```python
from build123d import *

# Parameters (mm, degrees)
CROQUIS1_W              = 16
CROQUIS1_H              = 23
SALIENTE_EXTRUIR1_DEPTH = 2
CROQUIS2_W              = 13
CROQUIS2_H              = 20
SALIENTE_EXTRUIR2_DEPTH = 10
SALIENTE_EXTRUIR3_DEPTH = 6.5
CROQUIS4_R              = 2
CROQUIS4_R_2            = 1.5
CROQUIS4_W              = 4
CROQUIS4_H              = 1
CORTAR_EXTRUIR1_DEPTH   = 0.6
SALIENTE_EXTRUIR6_DEPTH = 6.5
REDONDEO1_R             = 0.5
CROQUIS6_R              = 0.75
SALIENTE_EXTRUIR7_DEPTH = 0.25
MATRIZL1_COUNT          = 2
MATRIZL1_PITCH          = 6.666666667
MATRIZL2_COUNT          = 2
MATRIZL2_PITCH          = 6.666666667


with BuildPart() as part:
    # Croquis1 → Saliente-Extruir1 (new body)
    with BuildSketch(Plane(origin=(0, 0, 0), x_dir=(1, 0, 0), z_dir=(0, 1, 0))):
        Rectangle(CROQUIS1_W, CROQUIS1_H)
    extrude(amount=SALIENTE_EXTRUIR1_DEPTH)

    # Croquis2 → Saliente-Extruir2 (add)
    with BuildSketch(Plane.XZ):
        Rectangle(CROQUIS2_W, CROQUIS2_H)
    extrude(amount=SALIENTE_EXTRUIR2_DEPTH)

    # Croquis3 → Saliente-Extruir3 (add, symmetric)
    with BuildSketch(Plane(origin=(0, 0, 0), x_dir=(0, 0, -1), z_dir=(1, 0, 0))):
        with BuildLine():
            Line((8.5, 2), (-8.5, 2))
            Line((-8.5, 2), (-0.603629693, 3.914367561))
            ThreePointArc((-0.603629693, 3.914367561), (0.234425411, 4.156697965), (1.048170976, 4.471147542))
            Line((1.048170976, 4.471147542), (5.618369194, 6.470445319))
            ThreePointArc((5.618369194, 6.470445319), (5.795753126, 6.511830798), (5.976190969, 6.486930957))
            Line((5.976190969, 6.486930957), (6.048439126, 6.462964543))
            ThreePointArc((6.048439126, 6.462964543), (7.345603515, 5.609203874), (8.042100494, 4.221243251))
            Line((8.042100494, 4.221243251), (8.5, 2))
        make_face()
    extrude(amount=SALIENTE_EXTRUIR3_DEPTH, both=True)

    # Croquis4 → Cortar-Extruir1 (cut)
    with BuildSketch(Plane(origin=(0, 4.265025315, 1.351360717), x_dir=(1, 0, 0), z_dir=(0, 0.95329272, 0.302047992))):
        with Locations((0, 4)):
            Circle(CROQUIS4_R)
        with Locations((0, 4)):
            Circle(CROQUIS4_R_2, mode=Mode.SUBTRACT)
        with Locations((0, -4)):
            Rectangle(CROQUIS4_W, CROQUIS4_H)
    extrude(amount=-CORTAR_EXTRUIR1_DEPTH, mode=Mode.SUBTRACT)

    # Croquis5 → Saliente-Extruir6 (add, symmetric)
    with BuildSketch(Plane(origin=(0, 0, 0), x_dir=(0, 0, -1), z_dir=(1, 0, 0))):
        Polygon((-10, -0.2), (-10.3, -0.2), (-10.3, -0.5), (-10.6, -0.5), (-10.6, -0.8), (-10.9, -0.8), (-10, -10), (-10, -8), (-10.6, -1.1), (-10.3, -1.1), (-10.3, -0.8), (-10, -0.8), align=None)
    saliente_extruir6 = extrude(amount=SALIENTE_EXTRUIR6_DEPTH, both=True)

    # Simetría2: Saliente-Extruir6 across plane
    add(saliente_extruir6.mirror(Plane.XY))

    # Redondeo1
    redondeo1_edges = [part.edges().sort_by_distance(p)[0] for p in [
        (-8, 1, -11.5),
        (8, 1, -11.5),
        (8, 1, 11.5),
        (-8, 1, 11.5),
    ]]
    fillet(redondeo1_edges, radius=REDONDEO1_R)

    # Croquis6 → Saliente-Extruir7 (add, symmetric)
    with BuildSketch(Plane.XY):
        with BuildLine():
            Line((2.5, -10), (-2.5, -10))
            Line((-2.5, -10), (-2.5, -15.826794919))
            ThreePointArc((-2.5, -15.826794919), (-2.459807621, -15.976794919), (-2.35, -16.08660254))
            Line((-2.35, -16.08660254), (-0.65, -17.068097998))
            ThreePointArc((-0.65, -17.068097998), (-0.540192379, -17.177905619), (-0.5, -17.327905619))
            Line((-0.5, -17.327905619), (-0.5, -17.354700538))
            ThreePointArc((-0.5, -17.354700538), (-0.412132034, -17.566832573), (-0.2, -17.654700538))
            Line((-0.2, -17.654700538), (0.2, -17.654700538))
            ThreePointArc((0.2, -17.654700538), (0.412132034, -17.566832573), (0.5, -17.354700538))
            Line((0.5, -17.354700538), (0.5, -17.327905619))
            ThreePointArc((0.5, -17.327905619), (0.540192379, -17.177905619), (0.65, -17.068097998))
            Line((0.65, -17.068097998), (2.35, -16.08660254))
            ThreePointArc((2.35, -16.08660254), (2.459807621, -15.976794919), (2.5, -15.826794919))
            Line((2.5, -15.826794919), (2.5, -10))
        make_face()
        with Locations((0, -15.154700538)):
            Circle(CROQUIS6_R, mode=Mode.SUBTRACT)
    saliente_extruir7 = extrude(amount=SALIENTE_EXTRUIR7_DEPTH, both=True)

    # MatrizL1: Saliente-Extruir7 ×2
    with Locations(*[(0, 0, -i * MATRIZL1_PITCH) for i in range(1, MATRIZL1_COUNT)]):
        add(saliente_extruir7)

    # MatrizL2: Saliente-Extruir7 ×2
    with Locations(*[(0, 0, i * MATRIZL2_PITCH) for i in range(1, MATRIZL2_COUNT)]):
        add(saliente_extruir7)


solid = part.part
```
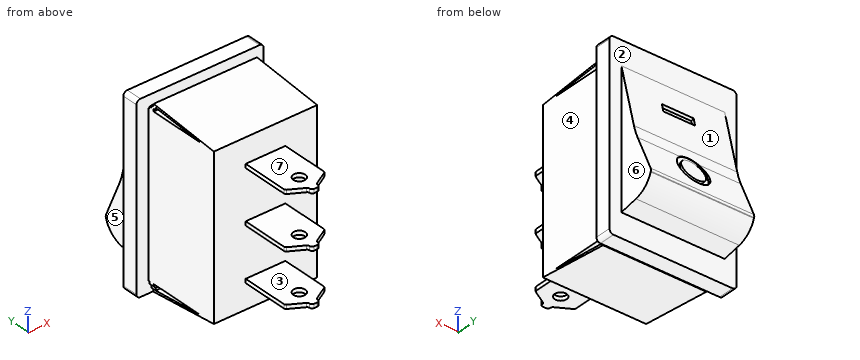
Check sheet for the modelled part. Datum: model origin and axes. Units: mm. Face numbers are marked on the shaded views. A direction names the side the tool comes from. Round coordinates to 2 decimals unless told otherwise and drop trailing zeros. Order: outer loops, then holes, each group sorted by start corner. A loop starts at its lowest first (then second) coordinate and runs counter-clockwise, first axis right, second up.
1) Go/stop test with flat-tipped pins: pin 1 Ø10 at (y, z) = (-8, -1) entering from -X; pin 2 Ø0.6 at (y, z) = (-14.5, 0) entering from +X; pin 3 Ø2 at (y, z) = (-12, 4.5) entering from +X; pin 4 Ø5 at (x, y) = (3.5, -11.5) entering from -Z. Record where each tip stops, or that it passes through.
2) Scan lines: line 1 (Z direction, x = 1.5, y = -11.75); line 2 (Y direction, x = 6.75, z = 3.25); line 3 (Z direction, x = -1.25, y = -5.75). Record each from-to range of solid material in increasing order.
3) Section check A-A (z = -9.25). Record the boundary of the cut face in (x, y).
4) Mould release check, pull along Z, two halves, no side actions. Record for the marked faces 1, 2 and 3: +Z half, -Z half, draft (parallel to the pull), parting line (faces both ways), or undercut.
5) Tool access check on the marked faces 4, 5, 6 and 7. Record the directions out of +Z, -Z, +X, -X, +Y, -Y that give a thin tool (end or side, any length) a straight path to the whole face; none if there is none.
Result:
1. pin 1: stops at x = -6.5
1. pin 2: stops at x = 2.5
1. pin 3: passes through
1. pin 4: stops at z = -10.1
2. line 1: z = -6.92 to -6.42, -0.25 to 0.25, 6.42 to 6.92
2. line 2: y = 0 to 2
2. line 3: z = -10.42 to -10.2, -10 to 10, 10.2 to 10.42
3. outline: (-8, 0) - (-6.5, 0) - (-6.5, -10) - (6.5, -10) - (6.5, 0) - (8, 0) - (8, 2) - (-8, 2) - close
4. face 1: +Z half
4. face 2: draft
4. face 3: undercut
5. face 4: +Z, -Z, +X, -Y
5. face 5: +Z, -Z, -X, +Y
5. face 6: +Z, -Z, +X, +Y
5. face 7: +Z, +X, -X, -Y
